Geometry check sheet. Reference: the model listing, model coordinates, mm. A direction names the side the tool comes from. Give positions to 0.01 mm unless a question says otherwise; leave off trailing zeros. Loops run counter-clockwise (first coordinate to the right, second up) from the corner with the lowest first, then second, coordinate; pieces in that order, holes last. Notation, with made-up numbers: (-39, -38) -> (-34, -38) arc R26 ccw to (-34, -7) -> close; hole circle Ø7 at (17.5, 51.5). An arc over 180 degrees is marked (long way). Answer as a JSON object with one key per item and string values.
from build123d import *

# Parameters (mm, degrees)
BOSS_EXTRUDE1_DEPTH                = 14
TAP_DRILL_FOR_M3X0_5_TAP1_D        = 2.5
TAP_DRILL_FOR_M3X0_5_TAP1_DEPTH    = 3
TAP_DRILL_FOR_M3X0_5_TAP1_TIP      = 0.751075774
CUT_EXTRUDE1_REACH                 = 5
SKETCH4_R                          = 3
TAP_DRILL_FOR_M2_5X0_45_TAP1_D     = 2.05
TAP_DRILL_FOR_M2_5X0_45_TAP1_DEPTH = 3


with BuildPart() as part:
    # Sketch1 → Boss-Extrude1 (new body)
    with BuildSketch(Plane(origin=(0, 0, 0), x_dir=(0, 0, -1), z_dir=(1, 0, 0))):
        with BuildLine():
            Line((0, 0), (10, 0))
            Line((10, 0), (10, 30))
            Line((10, 30), (7, 30))
            Line((7, 30), (7, 7))
            ThreePointArc((7, 7), (6.121320344, 4.878679656), (4, 4))
            Line((4, 4), (0, 4))
            Line((0, 4), (0, 0))
        make_face()
    extrude(amount=BOSS_EXTRUDE1_DEPTH)

    # Tap Drill for M3x0.5 Tap1
    with Locations(Plane(origin=(0, 0, 0), x_dir=(-1, 0, 0), z_dir=(0, -1, 0))):
        with Locations((-11, 7), (-3, 3)):
            Hole(TAP_DRILL_FOR_M3X0_5_TAP1_D / 2, depth=TAP_DRILL_FOR_M3X0_5_TAP1_DEPTH)
            with Locations((0, 0, -(TAP_DRILL_FOR_M3X0_5_TAP1_DEPTH + TAP_DRILL_FOR_M3X0_5_TAP1_TIP / 2))):  # 118° drill point
                Cone(0, TAP_DRILL_FOR_M3X0_5_TAP1_D / 2, TAP_DRILL_FOR_M3X0_5_TAP1_TIP, mode=Mode.SUBTRACT)

    # Sketch4 → Cut-Extrude1 (cut, up to next)
    with BuildSketch(Plane.XY.offset(-7), mode=Mode.PRIVATE) as cut_extrude1_sk1:
        with Locations((7, 17.85)):
            Circle(SKETCH4_R)
    cut_extrude1_tool1 = extrude(cut_extrude1_sk1.sketch, amount=-CUT_EXTRUDE1_REACH, mode=Mode.PRIVATE) & part.part
    add(cut_extrude1_tool1.solids().sort_by_distance((7, 17.85, -7))[0], mode=Mode.SUBTRACT)

    # Tap Drill for M2.5x0.45 Tap1
    with Locations(Plane.XY.offset(-7)):
        with Locations((1.737569913, 12.587569913), (12.262430087, 23.112430087)):
            Hole(TAP_DRILL_FOR_M2_5X0_45_TAP1_D / 2, depth=TAP_DRILL_FOR_M2_5X0_45_TAP1_DEPTH)


solid = part.part
1) Material ranges on line 1 along X through (y, z) = (1.8, -7); line 2 along Y through (x, z) = (7, -8.5); line 3 along Z through (x, y) = (11, 0.6), recorded low to high. Write a range as from..to.
Geometry check:
{"line 1": "x = 0..9.75, 12.25..14", "line 2": "y = 0..14.85, 20.85..30", "line 3": "z = -10..-8.25, -5.75..0"}
2) Draft check along Z on faces 1 (the face through (10.8, 3.62, -6.92)), 2 (the face through (0, 11.9, -7.2)), 3 (the face through (6.9, 4.9, -6.14)). Enter one of: pulls with the +Z half, pulls with the -Z half, needs draft (parallel to the pull), parting line crosses it, or undercut.
Geometry check:
{"face 1": "undercut", "face 2": "needs draft", "face 3": "pulls with the +Z half"}
3) Section check D-D on z = -8.75. Record the cut outline in (x, y) (3 decimals).
Geometry check:
{"outline": "(0, 0) -> (14, 0) -> (14, 30) -> (0, 30) -> close; hole circle Ø2.05 at (1.738, 12.588); hole circle Ø6 at (7, 17.85); hole circle Ø2.05 at (12.262, 23.112)"}
4) Section check A-A on x = 12.75. Record the cut outline in (y, z).
Geometry check:
{"outline": "(0, -10) -> (22.21, -10) -> (22.21, -7) -> (7, -7) arc R3 cw to (4, -4) -> (4, 0) -> (0, 0) -> close; (24.01, -10) -> (30, -10) -> (30, -7) -> (24.01, -7) -> close"}
5) Tool access check on faces 4 (the face through (7, 4, -2)), 5 (the face through (4.19, 1.52, -3.38)), 6 (the face through (14, 11.9, -7.2)). Record the directions out of +Z, -Z, +X, -X, +Y, -Y that give a thin tool (end or side, any length) a straight path to the whole face; none if there is none.
Geometry check:
{"face 4": "+Z, +X, -X, +Y", "face 5": "-Y", "face 6": "+Z, -Z, +X, +Y, -Y"}
6) Depth check by flat-ended pin: P1, Ø7, axis at x = 7, y = 17.85, coming from the +Z side; P2, Ø2, axis at x = 4, z = -3, coming from the +Y side; P3, Ø2, axis at x = 3, z = -3, coming from the -Y side; P4, Ø2.5, axis at x = 12.26, y = 23.11, coming from the -Z side. Enter the tip coordinate at first touch or a pass-through.
Geometry check:
{"P1": "stops at z = -7", "P2": "stops at y = 4", "P3": "stops at y = 3.15", "P4": "stops at z = -10"}
7) Section check C-C on y = 16.5. Record the cut outline in (x, z), plus the area to 3 significant figures.
Geometry check:
{"outline": "(0, -10) -> (4.32, -10) -> (4.32, -7) -> (0, -7) -> close; (9.68, -10) -> (14, -10) -> (14, -7) -> (9.68, -7) -> close", "area": "25.9 mm2"}
8) Section check B-B on y = 2.5. Record the cut outline in (x, z).
Geometry check:
{"outline": "(0, -10) -> (14, -10) -> (14, 0) -> (0, 0) -> close; hole circle Ø2.5 at (3, -3); hole circle Ø2.5 at (11, -7)"}
